Check sheet for the modelled part. Datum: model origin and axes. Units: mm. Face numbers are marked on the shaded views. Give positions to 0.01 mm unless a question says otherwise; leave off trailing zeros. Write each loop counter-clockwise with the first axis right and the second up, starting at its lowest first coordinate (ties: lowest second). Pieces come first, ordered by that corner, then holes.
from build123d import *

# Parameters (mm, degrees)
SKETCH_1_W                = 8
SKETCH_1_H                = 12
EXTRUDE_1_DEPTH           = 100
CUT_EXTRUDE_3_DEPTH       = 10
CUT_EXTRUDE_11_DEPTH      = 100
SKETCH_12_4_W             = 4
SKETCH_12_4_H             = 4.473349964
SKETCH_16_W               = 6.416978836
SKETCH_16_H               = 19.46348209
CUT_EXTRUDE_14_DEPTH      = 18
CUT_EXTRUDE_14_DEPTH_BACK = 18
SKETCH_17_W               = 1.2
SKETCH_17_H               = 11.2
CUT_EXTRUDE_15_DEPTH      = 3


with BuildPart() as part:
    # Sketch 1 → Extrude 1 (new body)
    with BuildSketch(Plane.XY):
        with Locations((-6.4060213, -18.331726276)):
            Rectangle(SKETCH_1_W, SKETCH_1_H)
    extrude(amount=EXTRUDE_1_DEPTH)

    # Sketch 5 → Cut-Extrude 3 (cut)
    with BuildSketch(Plane.ZY.offset(10.4060213)):
        with BuildLine():
            Line((7.555938676, -20.573863088), (7.555938676, -16.089589464))
            ThreePointArc((7.555938676, -16.089589464), (3.802125111, -15.149730715), (1.6, -18.331726276))
            ThreePointArc((1.6, -18.331726276), (3.802125111, -21.513721837), (7.555938676, -20.573863088))
        make_face()
    extrude(amount=-CUT_EXTRUDE_3_DEPTH, mode=Mode.SUBTRACT)

    # Sketch 2 → Cut-Extrude 11 (cut)
    with BuildSketch(Plane.ZY.offset(10.4060213)):
        with BuildLine():
            Line((100, -12.331726276), (-0.01185689, -12.331726276))
            Line((-0.01185689, -12.331726276), (-0.01185689, -24.331726276))
            Line((-0.01185689, -24.331726276), (22.555938676, -24.331726276))
            Line((22.555938676, -24.331726276), (100, -24.331726276))
            Line((100, -24.331726276), (100.024770408, -20.562939428))
            Line((100.024770408, -20.562939428), (8.52899758, -20.562939428))
            ThreePointArc((8.52899758, -20.562939428), (0.770675983, -18.338179262), (8.522124603, -16.089589464))
            Line((8.522124603, -16.089589464), (100.024770408, -16.089589464))
            Line((100.024770408, -16.089589464), (100, -12.331726276))
        make_face()
    extrude(amount=-CUT_EXTRUDE_11_DEPTH, mode=Mode.SUBTRACT)

    # Sketch 12 → Revolve 3 (revolve)
    with BuildSketch(Plane.XY.offset(100)):
        with BuildLine():
            Line((-6.4060213, -13.526264446), (-6.4060213, -12.726264446))
            ThreePointArc((-6.4060213, -12.726264446), (-12.0060213, -18.326264446), (-6.4060213, -23.926264446))
            Line((-6.4060213, -23.926264446), (-6.4060213, -23.126264446))
            ThreePointArc((-6.4060213, -23.126264446), (-11.2060213, -18.326264446), (-6.4060213, -13.526264446))
        make_face()
    revolve(axis=Axis((-6.4060213, -12.726264446, 100), (0, -1, 0)))

    # Sketch 12_4 → Cut-Revolve 1 (revolve, cut)
    with BuildSketch(Plane.XY.offset(100)):
        with Locations((-8.4060213, -18.326264446)):
            Rectangle(SKETCH_12_4_W, SKETCH_12_4_H)
        with BuildLine():
            Line((-6.4060213, -16.089589464), (-6.4060213, -13.526264446))
            ThreePointArc((-6.4060213, -13.526264446), (-11.2060213, -18.326264446), (-6.4060213, -23.126264446))
            Line((-6.4060213, -23.126264446), (-6.4060213, -20.562939428))
            Line((-6.4060213, -20.562939428), (-10.4060213, -20.562939428))
            Line((-10.4060213, -20.562939428), (-10.4060213, -16.089589464))
            Line((-10.4060213, -16.089589464), (-6.4060213, -16.089589464))
        make_face()
    revolve(axis=Axis((-6.4060213, -12.726264446, 100), (0, -1, 0)), mode=Mode.SUBTRACT)

    # Sketch 16 → Cut-Extrude 14 (cut, two sides)
    with BuildSketch(Plane(origin=(-52.372486851, 0, 30.237269382), x_dir=(0.5, 0, 0.866025404), z_dir=(-0.866025404, 0, 0.5))) as cut_extrude_14_sk:
        with Locations((89.420800734, -19.375704403)):
            Rectangle(SKETCH_16_W, SKETCH_16_H)
    extrude(amount=CUT_EXTRUDE_14_DEPTH, mode=Mode.SUBTRACT)
    extrude(cut_extrude_14_sk.sketch, amount=-CUT_EXTRUDE_14_DEPTH_BACK, mode=Mode.SUBTRACT)

    # Sketch 17 → Cut-Extrude 15 (cut)
    with BuildSketch(Plane(origin=(43.106155658, 0, 74.662051718), x_dir=(0.866025404, 0, -0.5), z_dir=(0.5, 0, 0.866025404))):
        with Locations((-55.537824976, -18.326264446)):
            Rectangle(SKETCH_17_W, SKETCH_17_H)
    extrude(amount=-CUT_EXTRUDE_15_DEPTH, mode=Mode.SUBTRACT)


solid = part.part
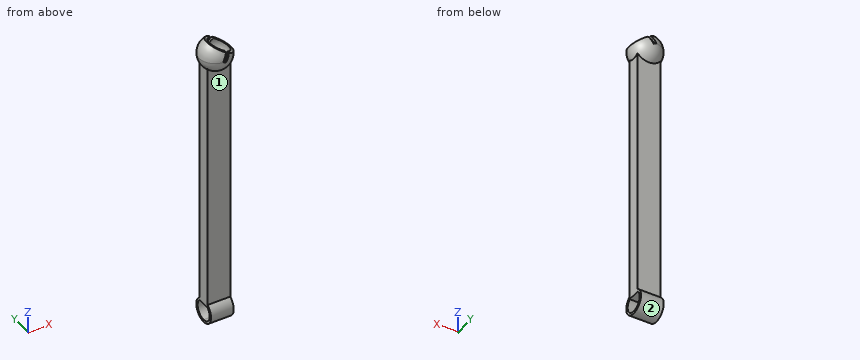
1) Draft check along Z on the marked faces 1 and 2. Enter one of: +Z half, -Z half, draft (parallel to the pull), parting line (faces both ways), or undercut.
2) Sectioned sample at B-B on z = 90. Record the boundary of the cut face in (x, y).
3) Gauge pin test, flat ends, axial feed: pin 1 (1.5 mm diameter, centred on x = -11, y = -18, fed in from -Z); pin 2 (2.5 mm diameter, centred on x = -8, z = 71.5, fed in from -Y); pin 3 (5 mm diameter, centred on x = -5, z = 78.5, fed in from +Y); pin 4 (6.5 mm diameter, centred on y = -20, z = 39.5, fed in from -X). Record the tip position at first contact, or that the pin passes through.
4) Scan lines: L1, parallel to Y at x = -9, z = 14; L2, parallel to Z at x = -8.5, y = -17.75; L3, parallel to X at y = -20.5, z = 13. Record each from-to range of solid material in increasing order.
5) Sectioned sample at A-A on y = -19.5. Record the boundary of the cut face in (x, z).
Answers below:
1. face 1: undercut
1. face 2: undercut
2. outline: (-10.41, -20.56) - (-2.41, -20.56) - (-2.41, -16.09) - (-10.41, -16.09) - close
3. pin 1: stops at z = 0.77
3. pin 2: stops at y = -20.56
3. pin 3: stops at y = -16.09
3. pin 4: stops at x = -10.41
4. L1: y = -20.56 to -16.09
4. L2: z = 0.81 to 1.65, 7.56 to 95.72, 104.28 to 104.46
4. L3: x = -10.41 to -2.41
5. outline: (-10.41, 0.94) - (-2.41, 0.94) - (-2.41, 1.81) - (-10.41, 1.81) - close; (-10.41, 7.56) - (-2.41, 7.56) - (-2.41, 96.26) arc R5.48 ccw to (-0.93, 100.09) - (-1.79, 100.58) arc R4.65 cw (long way) to (-8.21, 104.29) - (-9.07, 104.78) arc R5.48 ccw to (-10.41, 96.26) - close
